```python
from build123d import *

# Parameters (mm, degrees)
SKETCH1_R           = 26.19375
BOSS_EXTRUDE1_DEPTH = 22.225
SKETCH2_R           = 31.75
BOSS_EXTRUDE2_DEPTH = 6.35
SKETCH4_R           = 3.96875
BOSS_EXTRUDE3_DEPTH = 15.875


with BuildPart() as part:
    # Sketch1 → Boss-Extrude1 (new body)
    with BuildSketch(Plane(origin=(0, 0, 0), x_dir=(1, 0, 0), z_dir=(0, 1, 0))):
        Circle(SKETCH1_R)
    extrude(amount=BOSS_EXTRUDE1_DEPTH)

    # Sketch2 → Boss-Extrude2 (add)
    with BuildSketch(Plane(origin=(0, 22.225, 0), x_dir=(1, 0, 0), z_dir=(0, 1, 0))):
        Circle(SKETCH2_R)
    extrude(amount=-BOSS_EXTRUDE2_DEPTH)

    # Sketch3 → Revolve1 (revolve)
    with BuildSketch(Plane(origin=(0, 22.225, 0), x_dir=(1, 0, 0), z_dir=(0, 1, 0))):
        with BuildLine():
            Line((0, -12.7), (0, 12.7))
            ThreePointArc((0, 12.7), (12.7, 0), (0, -12.7))
        make_face()
    revolve(axis=Axis((0, 22.225, -45.379060403), (0, 0, 1)))

    # Sketch4 → Boss-Extrude3 (add)
    with BuildSketch(Plane.XZ):
        Circle(SKETCH4_R)
    extrude(amount=BOSS_EXTRUDE3_DEPTH)


solid = part.part
```
Design review of the part built by this model. Coordinates are the model's own, in mm. A direction names the side the tool comes from. Give positions to 0.01 mm unless a question says otherwise; leave off trailing zeros. Order: outer loops, then holes, each group sorted by start corner. A loop starts at its lowest first (then second) coordinate and runs counter-clockwise, first axis right, second up. Notation, with made-up numbers: (-33, 72) - (1, 72) arc R16 ccw to (1, 82) - close; hole circle Ø9 at (36.25, 7). An arc over 180 degrees is marked (long way). Use a Markdown table: item, result. Add a question column.
(1) Machinability: for faces 1 (the face through (5, 15.875, -26)), 2 (the face through (14, 22.225, 0)), 3 (the face through (0, -15.875, 0)), which of the approach directions +Z, -Z, +X, -X, +Y, -Y give a long, thin tool a straight path to every point of the face, cutting with its end or side? Answer none if there is none.
(2) Add section D-D on x = 7. Give the boundary of the cut face in (y, z) (3 decimals).
(3) Add section A-A on z = 0. Give the boundary of the cut face in (x, y) (3 decimals), then the cut area to 3 significant figures.
(4) Add section C-C on y = -5. Give the boundary of the cut face in (x, z), then the cut area to 3 significant figures.
(5) Clearance check with flat-ended pins moving along their axes: P1, Ø4, axis at y = 18.5, z = 16.5, coming from the -X side; P2, Ø4, axis at y = 19, z = -25, coming from the -X side; P3, Ø6, axis at x = 0.5, y = 18, coming from the -Z side. State where each tip first meets the part, or that it passes through.
(6) Add section B-B on x = -5.5. Give the boundary of the cut face in (y, z) (3 decimals), then the cut area to 3 significant figures.
(7) Wall thickness on probe 1 along Y at (x, z) = (-5, 12) (3 decimals); probe 2 along Y at (x, z) = (-23.5, 12) (3 decimals); probe 3 along Z at (x, y) = (-12, 9): over which ranges is each line inside the solid? List them lowest first. Write a range as [from, to].
Report:
| question | item | result |
|---|---|---|
| 1 | face 1 | -Y |
| 1 | face 2 | +Y |
| 1 | face 3 | +Z, -Z, +X, -X, -Y |
| 2 | outline | (0, -25.241) - (15.875, -25.241) - (15.875, -30.969) - (22.225, -30.969) - (22.225, -10.597) arc R10.597 ccw to (22.225, 10.597) - (22.225, 30.969) - (15.875, 30.969) - (15.875, 25.241) - (0, 25.241) - close |
| 3 | outline | (-31.75, 15.875) - (-26.194, 15.875) - (-26.194, 0) - (-3.969, 0) - (-3.969, -15.875) - (3.969, -15.875) - (3.969, 0) - (26.194, 0) - (26.194, 15.875) - (31.75, 15.875) - (31.75, 22.225) - (12.7, 22.225) arc R12.7 ccw to (-12.7, 22.225) - (-31.75, 22.225) - close |
| 3 | area | 1,610 mm² |
| 4 | outline | circle Ø7.94 at (0, 0) |
| 4 | area | 49.5 mm² |
| 5 | P1 | stops at x = -28.25 |
| 5 | P2 | stops at x = -21.89 |
| 5 | P3 | stops at z = -31.75 |
| 6 | outline | (0, -25.61) - (15.875, -25.61) - (15.875, -31.27) - (22.225, -31.27) - (22.225, -11.447) arc R11.447 ccw to (22.225, 11.447) - (22.225, 31.27) - (15.875, 31.27) - (15.875, 25.61) - (0, 25.61) - close |
| 6 | area | 1,420 mm² |
| 7 | probe 1 | y = [0, 22.225] |
| 7 | probe 2 | y = [15.875, 22.225] |
| 7 | probe 3 | z = [-23.28, 23.28] |
